from build123d import *

# Parameters (mm, degrees)
F0_R           = 21.5
F1_DEPTH       = 40
F3_R           = 15
F1_FACE_R      = 21.5
F6_D           = 9
F6_CBORE_D     = 14.25
F6_CBORE_DEPTH = 8
F7_R           = 2


with BuildPart() as f1:
    # F0 (on Front) → F1 (new body)
    with BuildSketch(Plane.XZ):
        Circle(F0_R)
    extrude(amount=F1_DEPTH)

    # F3 (on offset) → F4 section 0
    with BuildSketch(Plane.XZ.offset(56)):
        Circle(F3_R)
    # F1_face (on face) → F4 section 1
    with BuildSketch(Plane.XZ.offset(40)):
        Circle(F1_FACE_R)
    loft()

    # F6 (through all)
    with Locations(Plane.XZ.offset(56)):
        with Locations((0, 0)):
            CounterBoreHole(F6_D / 2, F6_CBORE_D / 2, F6_CBORE_DEPTH)

    # F7
    f7_edges = [f1.edges().sort_by_distance(p)[0] for p in [
        (-21.5, -40, 0),
        (-15, -56, 0),
    ]]
    fillet(f7_edges, radius=F7_R)


solid = f1.part
Design review of the part built by this model. Coordinates are the model's own, in mm. A direction names the side the tool comes from. Round coordinates to 2 decimals unless told otherwise and drop trailing zeros. Loops run counter-clockwise (first coordinate to the right, second up) from the corner with the lowest first, then second, coordinate; pieces in that order, holes last. Notation, with made-up numbers: (-34, -1) -> (-16, -1) arc R13 cw to (-16, 22) -> close; hole circle Ø10 at (-26, 65.25). An arc over 180 degrees is marked (long way). Use one line per item in the form item = value. Start each with the question number.
Q1. Draft analysis for pull direction Z (two halves, no side actions). For faces 1 (the face through (6.58, -52.06, -2.73)), 2 (the face through (-2.799, -19.527, 21.317)), 3 (the face through (0, 0, 5)), state which applies: +Z half, -Z half, draft (parallel to the pull), parting line (faces both ways), or undercut.
Q2. Machinability: for faces 4 (the face through (0, -48, -5)), 5 (the face through (0.59, -23.66, 4.46)), which of the approach directions +Z, -Z, +X, -X, +Y, -Y give a long, thin tool a straight path to every point of the face, cutting with its end or side? Answer none if there is none.
Q3. We need section A-A on y = -33. Give the boundary of the cut face in (x, z).
Q4. For pin 1 Ø1 at (x, z) = (7, -0.5) entering from +Y; pin 2 Ø1.5 at (x, z) = (-12, -11.5) entering from -Y; pin 3 Ø1 at (x, y) = (-15.5, -18.5) entering from -Z; pin 4 Ø1.5 at (y, z) = (-27.5, -12) entering from -X, all flat-tipped, find the tip position at first contact; note any pin that passes through.
Q5. We need section B-B on y = -42.5. Give the boundary of the cut face in (x, z), then the cut area to 3 significant figures.
Q6. Wall thickness on line 1 along Z through (x, y) = (0, -21.5); line 2 along X through (y, z) = (-33, -1); line 3 along Z through (x, y) = (0, -50) (1 decimal): over which ranges is each line inside the solid? List them lowest first. Write a range as [from, to].
Calculated:
q1.face_1 = undercut
q1.face_2 = parting line
q1.face_3 = draft
q2.face_4 = -Y
q2.face_5 = +Y, -Y
q3.outline = circle Ø43 at (0, 0); hole circle Ø9 at (0, 0)
q4.pin_1 = 0
q4.pin_2 = -53.86
q4.pin_3 = -15.4
q4.pin_4 = -18.32
q5.outline = circle Ø40.97 at (0, 0); hole circle Ø9 at (0, 0)
q5.area = 1,250 mm²
q6.line_1 = [-21.5, -4.5], [4.5, 21.5]
q6.line_2 = [-21.48, -4.39], [4.39, 21.48]
q6.line_3 = [-17.4, -7.1], [7.1, 17.4]
